from build123d import *

# Parameters (mm, degrees)
F1_DEPTH = 3
F2_R     = 0.7


with BuildPart() as f1:
    # F0 (on Top) → F1 (new body)
    with BuildSketch(Plane.XY):
        with BuildLine():
            ThreePointArc((37.675, 25.6), (36.79632, 27.72132), (34.675, 28.6))
            Line((34.675, 28.6), (-34.675, 28.6))
            ThreePointArc((-34.675, 28.6), (-36.79632, 27.72132), (-37.675, 25.6))
            Line((-37.675, 25.6), (-37.675, -25.6))
            ThreePointArc((-37.675, -25.6), (-36.79632, -27.72132), (-34.675, -28.6))
            Line((-34.675, -28.6), (26.675, -28.6))
            ThreePointArc((26.675, -28.6), (34.453175, -25.378175), (37.675, -17.6))
            Line((37.675, -17.6), (37.675, 25.6))
        make_face()
        with BuildLine():
            ThreePointArc((34.675, 26.6), (35.382107, 26.307107), (35.675, 25.6))
            Line((35.675, 25.6), (35.675, -17.6))
            ThreePointArc((35.675, -17.6), (33.038961, -23.963961), (26.675, -26.6))
            Line((26.675, -26.6), (-34.675, -26.6))
            ThreePointArc((-34.675, -26.6), (-35.382107, -26.307107), (-35.675, -25.6))
            Line((-35.675, -25.6), (-35.675, 25.6))
            ThreePointArc((-35.675, 25.6), (-35.382107, 26.307107), (-34.675, 26.6))
            Line((-34.675, 26.6), (34.675, 26.6))
        make_face(mode=Mode.SUBTRACT)
    extrude(amount=F1_DEPTH)

    # F2
    f2_edges = [f1.edges().sort_by_distance(p)[0] for p in [
        (-37.675, 0, 0),
        (0, 26.6, 3),
        (-35.675, 0, 3),
        (35.675, 4, 3),
    ]]
    fillet(f2_edges, radius=F2_R)


solid = f1.part
Design review of the part built by this model. Coordinates are the model's own, in mm. A direction names the side the tool comes from. Round coordinates to 2 decimals unless told otherwise and drop trailing zeros. Write each loop counter-clockwise with the first axis right and the second up, starting at its lowest first coordinate (ties: lowest second). Pieces come first, ordered by that corner, then holes. Notation, with made-up numbers: (18, 50) -> (69, 50) arc R11 cw to (69, 68) -> close; hole circle Ø8 at (87, 44.5). An arc over 180 degrees is marked (long way). One line per item, written item: value. Start each with the question number.
Q1. Add section B-B (y = 7.5). Give the boundary of the cut face in (x, z) (3 decimals), then the cut area to 3 significant figures.
Q2. Add section C-C (z = 1.65). Give the boundary of the cut face in (x, y) (3 decimals).
Q3. The part is to be moulded in two halves that separate along Y. For faces 3 (the face through (-37.675, 0, 2)), 4 (the face through (35.675, 4, 1)), 5 (the face through (-36.773, 27.745, 1.834)), say which applies: pulls with the +Y half, pulls with the -Y half, needs draft (parallel to the pull), parting line crosses it, or undercut.
Q4. To check wall thickness, follow probe 1 along X at (y, z) = (-5, 0.6) (3 decimals); probe 2 along Y at (x, z) = (13, 2.2); probe 3 along Y at (x, z) = (19.5, 2.65). State the ranges of each line that lie inside material, in increasing order.
Q5. Insertion check: P1, Ø1.5, axis at y = -19, z = 1.5, coming from the +X side; P2, Ø12, axis at x = -28, y = 17.5, coming from the +Z side. Each pin has a flat end and moves straight along its axis. Give the tip position at first contact, or say it passes through.
Q6. Add section A-A (x = 3). Give the boundary of the cut face in (y, z).
Q7. Tool access review of faces 1 (the face through (37.675, 4, 2)), 2 (the face through (0, 26.6, 1)): name each direction out of +Z, -Z, +X, -X, +Y, -Y from which nothing blocks a thin tool from reaching the whole face with its end or side.
Response:
1. outline: (-37.675, 0.7) arc R0.7 ccw to (-36.975, 0) -> (-35.675, 0) -> (-35.675, 2.3) arc R0.7 ccw to (-36.375, 3) -> (-37.675, 3) -> close; (35.675, 0) -> (36.975, 0) arc R0.7 ccw to (37.675, 0.7) -> (37.675, 3) -> (36.375, 3) arc R0.7 ccw to (35.675, 2.3) -> close
1. area: 11.6 mm^2
2. outline: (-37.675, -25.6) arc R3 ccw to (-34.675, -28.6) -> (26.675, -28.6) arc R11 ccw to (37.675, -17.6) -> (37.675, 25.6) arc R3 ccw to (34.675, 28.6) -> (-34.675, 28.6) arc R3 ccw to (-37.675, 25.6) -> close; hole (-35.675, -25.6) arc R1 ccw to (-34.675, -26.6) -> (26.675, -26.6) arc R9 ccw to (35.675, -17.6) -> (35.675, 25.6) arc R1 ccw to (34.675, 26.6) -> (-34.675, 26.6) arc R1 ccw to (-35.675, 25.6) -> close
3. face 3: needs draft
3. face 4: undercut
3. face 5: pulls with the +Y half
4. probe 1: x = -37.668 to -35.675, 35.675 to 37.668
4. probe 2: y = -28.6 to -26.6, 26.6 to 28.6
4. probe 3: y = -28.6 to -26.69, 26.69 to 28.6
5. P1: stops at x = 37.66
5. P2: passes through
6. outline: (-28.6, 0.7) arc R0.7 ccw to (-27.9, 0) -> (-26.6, 0) -> (-26.6, 2.3) arc R0.7 ccw to (-27.3, 3) -> (-28.6, 3) -> close; (26.6, 0) -> (27.9, 0) arc R0.7 ccw to (28.6, 0.7) -> (28.6, 3) -> (27.3, 3) arc R0.7 ccw to (26.6, 2.3) -> close
7. face 1: +Z, -Z, +X, +Y, -Y
7. face 2: +Z, -Z
